```python
from build123d import *

# Parameters (mm, degrees)
SKETCH1_R          = 2.8
SKETCH1_R_2        = 8
BASE_FLANGE1_DEPTH = 2


# Sheet-metal steps are written as plain solids
with BuildPart() as part:
    # Sketch1 → Base-Flange1 (new body)
    with BuildSketch(Plane(origin=(0, 0, 0), x_dir=(1, 0, 0), z_dir=(0, 1, 0))):
        Polygon((-90, 91.5), (90, 91.5), (90, -91.5), (-90, -91.5), (-90, -47), (-128, -47), (-128, 47), (-90, 47), align=None)
        with Locations(Location((-83, 55.0037, 0), (0, 0, 270))):
            Circle(SKETCH1_R, mode=Mode.SUBTRACT)
        with Locations(Location((-83, -55.0037, 0), (0, 0, 270))):
            Circle(SKETCH1_R, mode=Mode.SUBTRACT)
        with Locations(Location((75.76, -55.0037, 0), (0, 0, 270))):
            Circle(SKETCH1_R, mode=Mode.SUBTRACT)
        with Locations(Location((75.76, 55.0037, 0), (0, 0, 270))):
            Circle(SKETCH1_R, mode=Mode.SUBTRACT)
        with Locations(Location((-113, 31, 0), (0, 0, 270))):
            Circle(SKETCH1_R_2, mode=Mode.SUBTRACT)
        with Locations(Location((-113, -31, 0), (0, 0, 270))):
            Circle(SKETCH1_R_2, mode=Mode.SUBTRACT)
    extrude(amount=-BASE_FLANGE1_DEPTH)


solid = part.part
```
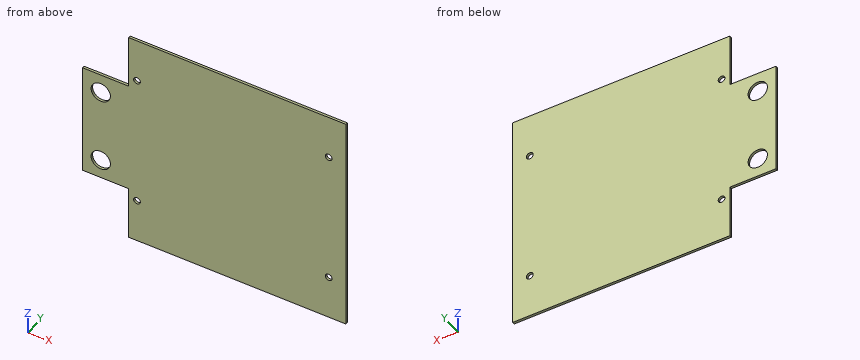
The model under review builds one solid part; all positions refer to its coordinate system, in mm. Round coordinates to 2 decimals unless told otherwise and drop trailing zeros. Loops run counter-clockwise (first coordinate to the right, second up) from the corner with the lowest first, then second, coordinate; pieces in that order, holes last. Notation, with made-up numbers: (75, 31.5) - (121, 31.5) arc R11 cw to (121, 49.5) - close; hole circle Ø6 at (20, 52). An arc over 180 degrees is marked (long way). Use a Markdown table: item, result. Add a question column.
Q1. Add section A-A (x = -113). State the section outline as (y, z) points.
Q2. For probe 1 along Z at (x, y) = (76, -0.3); probe 2 along Z at (x, y) = (-81.5, -0.8); probe 3 along X at (y, z) = (-1.45, 63), list the stretches that pass through material, from the lowest coordinate up.
Q3. Insertion check: pin 1 Ø1 at (x, y) = (-109, -0.5) entering from +Z; pin 2 Ø0.6 at (y, z) = (-1, 71.5) entering from -X. Each pin has a flat end and moves straight along its axis. Give the tip position at first contact, or say it passes through.
Q4. Add section D-D (x = -83). State the section outline as (y, z) points.
Q5. Add section B-B (y = -1.6). State the section outline as (x, z) points.
Q6. Add section C-C (z = 31). State the section outline as (x, y) points, plus the area to 3 significant figures.
Worked answers:
| question | item | result |
|---|---|---|
| 1 | outline | (-2, -47) - (0, -47) - (0, -39) - (-2, -39) - close; (-2, -23) - (0, -23) - (0, 23) - (-2, 23) - close; (-2, 39) - (0, 39) - (0, 47) - (-2, 47) - close |
| 2 | probe 1 | -91.5 to -57.79, -52.21 to 52.21, 57.79 to 91.5 |
| 2 | probe 2 | -91.5 to -57.37, -52.64 to 52.64, 57.37 to 91.5 |
| 2 | probe 3 | -90 to 90 |
| 3 | pin 1 | z = 47 |
| 3 | pin 2 | x = -90 |
| 4 | outline | (-2, -91.5) - (0, -91.5) - (0, -57.8) - (-2, -57.8) - close; (-2, -52.2) - (0, -52.2) - (0, 52.2) - (-2, 52.2) - close; (-2, 57.8) - (0, 57.8) - (0, 91.5) - (-2, 91.5) - close |
| 5 | outline | (-128, -47) - (-90, -47) - (-90, -91.5) - (90, -91.5) - (90, 91.5) - (-90, 91.5) - (-90, 47) - (-128, 47) - close; hole circle Ø16 at (-113, -31); hole circle Ø16 at (-113, 31); hole circle Ø5.6 at (-83, -55); hole circle Ø5.6 at (-83, 55); hole circle Ø5.6 at (75.76, -55); hole circle Ø5.6 at (75.76, 55) |
| 6 | outline | (-128, -2) - (-121, -2) - (-121, 0) - (-128, 0) - close; (-105, -2) - (90, -2) - (90, 0) - (-105, 0) - close |
| 6 | area | 404 mm² |
